CAD build for the part. Positions are in the model's coordinates, mm. A direction names the side the tool comes from. Give positions to 0.01 mm unless a question says otherwise; leave off trailing zeros. Order: outer loops, then holes, each group sorted by start corner. A loop starts at its lowest first (then second) coordinate and runs counter-clockwise, first axis right, second up.
Item 1: Band-saw the part on B-B on z = 68.5. Give the cut face in (x, y), plus the area to 3 significant figures.
Item 2: Band-saw the part on A-A on x = -23.5. Give the cut face in (y, z).
Item 3: Two-plate mould, pull along Y, no slides. Class faces 6 (the flat face through (75, -261, 74)), 7 (the flat face through (-1, 165, 135)), 8 (the flat face through (65.14, 675.37, 73.95)): released by +Y, released by -Y, zero draft, split by the parting line, or undercut.
Item 4: Flat gauge pins, fed straight in: P1, Ø6, axis at x = 29.5, y = -137, coming from the +Z side; P2, Ø4, axis at x = 58.5, z = 49, coming from the +Y side; P3, Ø1.5, axis at x = -62, z = 67.5, coming from the +Y side. Where does each tip first touch, or does it go through?
Item 5: Wall check: L1, parallel to X at y = -140, z = 33; L2, parallel to Z at x = 40, y = -68.5; L3, parallel to Y at x = -67, z = 81. Give the ranges that are in metal, low to high.
Item 6: Which spindle directions (+Z, -Z, +X, -X, +Y, -Y) get a long thin tool onto all of the face, cutting with end or side? Do faces 1 (the flat face through (62, -144.49, 75)), 2 (the flat face through (-62, 465.51, 80)), 3 (the flat face through (60, 165, 76)), 4 (the flat face through (-60, 164, 74)), 5 (the flat face through (-1, 165, 15)). Say none if no direction does.
Item 7: Band-saw the part on C-C on y = 230. Give the cut face in (x, z).
```python
from build123d import *

# Parameters (mm, degrees)
ESQUISSE1_W             = 75
ESQUISSE1_H             = 1050
BOSS_EXTRU_2_DEPTH      = 150
ESQUISSE2_W             = 226.933426854
ESQUISSE2_H             = 610
ENL_V_MAT_EXTRU_1_DEPTH = 15
ESQUISSE3_W             = 179.782352086
ESQUISSE3_H             = 610.96446809
ENL_V_MAT_EXTRU_2_DEPTH = 15
ESQUISSE4_W             = 199.341724475
ESQUISSE4_H             = 610
ENL_V_MAT_EXTRU_3_DEPTH = 15
ESQUISSE5_W             = 150
ESQUISSE5_H             = 610
ENL_V_MAT_EXTRU_4_DEPTH = 15
CHANFREIN1_SIZE         = 20
CHANFREIN2_SIZE         = 10
CHANFREIN3_SIZE         = 10


with BuildPart() as part:
    # Esquisse1 → Boss.-Extru.2 (new body)
    with BuildSketch(Plane.XY):
        with Locations((-37.5, 160.509714461)):
            Rectangle(ESQUISSE1_W, ESQUISSE1_H)
    boss_extru_2 = extrude(amount=BOSS_EXTRU_2_DEPTH)

    # Symétrie1: Boss.-Extru.2 across plane
    add(boss_extru_2.mirror(Plane(origin=(0, 685.509714461, 150), x_dir=(0, 0, 1), z_dir=(-1, 0, 0))))

    # Esquisse2 → Enlèv. mat.-Extru.1 (cut)
    with BuildSketch(Plane.XY):
        with Locations((0, 160.509714461)):
            Rectangle(ESQUISSE2_W, ESQUISSE2_H)
    extrude(amount=ENL_V_MAT_EXTRU_1_DEPTH, mode=Mode.SUBTRACT)

    # Esquisse3 → Enlèv. mat.-Extru.2 (cut)
    with BuildSketch(Plane.ZY.offset(75)):
        with Locations((89.891176043, 160.027480416)):
            Rectangle(ESQUISSE3_W, ESQUISSE3_H)
    extrude(amount=-ENL_V_MAT_EXTRU_2_DEPTH, mode=Mode.SUBTRACT)

    # Esquisse4 → Enlèv. mat.-Extru.3 (cut)
    with BuildSketch(Plane(origin=(75, 0, 0), x_dir=(0, 0, -1), z_dir=(1, 0, 0))):
        with Locations((-99.670862238, 160.509714461)):
            Rectangle(ESQUISSE4_W, ESQUISSE4_H)
    extrude(amount=-ENL_V_MAT_EXTRU_3_DEPTH, mode=Mode.SUBTRACT)

    # Esquisse5 → Enlèv. mat.-Extru.4 (cut)
    with BuildSketch(Plane.XY.offset(150)):
        with Locations((0, 160.509714461)):
            Rectangle(ESQUISSE5_W, ESQUISSE5_H)
    extrude(amount=-ENL_V_MAT_EXTRU_4_DEPTH, mode=Mode.SUBTRACT)

    # Chanfrein1
    chanfrein1_edges = [part.edges().sort_by_distance(p)[0] for p in [
        (75, 685.509714461, 75),
        (0, 685.509714461, 0),
        (0, 685.509714461, 150),
        (-75, 685.509714461, 75),
    ]]
    chamfer(chanfrein1_edges, length=CHANFREIN1_SIZE)

    # Chanfrein2
    chanfrein2_edges = [part.edges().sort_by_distance(p)[0] for p in [
        (75, 465.509714461, 75),
        (0, 465.509714461, 0),
        (-75, 465.509714461, 75),
        (0, 465.509714461, 150),
    ]]
    chamfer(chanfrein2_edges, length=CHANFREIN2_SIZE)

    # Chanfrein3
    # the kernel refuses this chamfer: 10 mm, written as the material it takes off along each edge
    with BuildSketch(Plane(origin=(-75, -145.454753629, 175.71682988), x_dir=(0.9996219169112968, 0.0274958766105877, 0), z_dir=(0, 0, -1))) as chanfrein3_piece_1:
        Polygon((CHANFREIN3_SIZE * 0.999621916911, CHANFREIN3_SIZE * 0.0274958766106), (-CHANFREIN3_SIZE * 0.0274958766106, CHANFREIN3_SIZE * 0.999621916911), (0, 0), align=None)
    extrude(amount=201.433659759, mode=Mode.SUBTRACT)
    with BuildSketch(Plane(origin=(-85.71682988, -144.490285539, 150), x_dir=(0, 0.027495876610587663, -0.9996219169112968), z_dir=(1, 0, 0)), Plane(origin=(100.71682988, -144.490285539, 0), x_dir=(0, 0.0274958766105877, 0.9996219169112968), z_dir=(-1, 0, 0))) as chanfrein3_piece_2:
        Polygon((CHANFREIN3_SIZE * 0.999621916911, -CHANFREIN3_SIZE * 0.0274958766106), (-CHANFREIN3_SIZE * 0.0274958766106, -CHANFREIN3_SIZE * 0.999621916911), (0, 0), align=None)
    extrude(amount=186.433659759, mode=Mode.SUBTRACT)
    with BuildSketch(Plane(origin=(75, -144.490285539, 175.71682988), x_dir=(-0.9996219169112968, 0.0274958766105877, 0), z_dir=(0, 0, -1))) as chanfrein3_piece_3:
        Polygon((CHANFREIN3_SIZE * 0.999621916911, -CHANFREIN3_SIZE * 0.0274958766106), (-CHANFREIN3_SIZE * 0.0274958766106, -CHANFREIN3_SIZE * 0.999621916911), (0, 0), align=None)
    extrude(amount=201.433659759, mode=Mode.SUBTRACT)


solid = part.part
```
The answers:
1. outline: (-75, -364.49) - (75, -364.49) - (75, -154.49) - (65, -144.49) - (60, -144.49) - (60, 465.51) - (65, 465.51) - (75, 475.51) - (75, 665.51) - (55, 685.51) - (-55, 685.51) - (-75, 665.51) - (-75, 475.51) - (-65, 465.51) - (-60, 465.51) - (-60, -145.45) - (-65, -145.45) - (-75, -155.45) - close
1. area: 139,000 mm2
2. outline: (-364.49, 0) - (-154.49, 0) - (-144.49, 10) - (-144.49, 15) - (465.51, 15) - (465.51, 10) - (475.51, 0) - (665.51, 0) - (685.51, 20) - (685.51, 130) - (665.51, 150) - (475.51, 150) - (465.51, 140) - (465.51, 135) - (-144.49, 135) - (-144.49, 140) - (-154.49, 150) - (-364.49, 150) - close
3. face 6: zero draft
3. face 7: undercut
3. face 8: released by +Y
4. P1: stops at z = 135
4. P2: stops at y = 684.01
4. P3: stops at y = 679.26
5. L1: x = -60 to 60
5. L2: z = 15 to 135
5. L3: y = -364.49 to -147.45, 467.51 to 673.51
6. face 1: +X
6. face 2: none
6. face 3: +Z, -Z, +X
6. face 4: +Z, -Z, -X
6. face 5: -Z, +X, -X
7. outline: (-60, 15) - (60, 15) - (60, 135) - (-60, 135) - close
